Read the model definition and answer for the solid it produces. Units are mm, in the model's axes. A direction names the side the tool comes from. Coordinates: 2 decimals unless noted, no trailing zeros. Write each loop counter-clockwise with the first axis right and the second up, starting at its lowest first coordinate (ties: lowest second). Pieces come first, ordered by that corner, then holes.
Item 1: Section C-C (z = -1.75) is taken. Give the vertices of the cut face in (x, y), then the cut area to 3 significant figures.
Item 2: Section A-A (y = -8.8) is taken. Give the vertices of the cut face in (x, z).
Item 3: Section B-B (x = -16) is taken. Give the vertices of the cut face in (y, z), then the cut area to 3 significant figures.
Item 4: A tool of negligible diameter and unlimited length cuts with its end or side. For faces 4 (the face through (-10.964, -8, 4)), 5 (the face through (-28, -8, 0.2)), 6 (the face through (-22.964, -8, -3)), 7 (the face through (-20, -10.457, -3)), 8 (the face through (-20, -6.257, -3)), from which of +Z, -Z, +X, -X, +Y, -Y can it reach the whole face along a straight path? Write none if from no direction.
Item 5: Straight lines are drawn through the part: probe 1 along X at (y, z) = (-8.3, 6.75); probe 2 along X at (y, z) = (-6.75, -2.5); probe 3 along Z at (x, y) = (-17.5, -7.2). For each, find the intervals that lie inside material, in ascending order.
Item 6: Each of these flat-tipped pins is pushed along its axis until it touches: P1, Ø2, axis at x = -9.5, y = -8, coming from the +Z side; P2, Ø2, axis at y = -7.5, z = -3, coming from the +X side; P3, Ø4, axis at x = -21.5, z = -1.5, coming from the -Y side; P4, Ø3, axis at y = -7.5, z = 4, coming from the +X side. Where does it stop, or does it pass through?
Item 7: Section D-D (x = -20.5) is taken. Give the vertices of the cut face in (y, z), then the cut area to 3 significant figures.
Item 8: Determine the mould class of faces 1 (the face through (-16, -8, 0.2)), 2 (the face through (-25.964, -8, 4)), 3 (the face through (-9, -8, 0.2)) for opening direction X: released by +X, released by -X, zero draft, split by the parting line, or undercut.
from build123d import *

# Parameters (mm, degrees)
F0_W     = 23
F0_H     = 6
F1_DEPTH = 0.2
F2_W     = 15
F2_H     = 6
F3_DEPTH = 7
F4_W     = 9
F4_H     = 4.2
F5_DEPTH = 0.2
F6_W     = 5
F6_H     = 4.2
F7_DEPTH = 5.3


with BuildPart() as f1:
    # F0 (on Top) → F1 (new body)
    with BuildSketch(Plane.XY):
        with Locations((-18.463512, -8.357231)):
            Rectangle(F0_W, F0_H)
    extrude(amount=F1_DEPTH)

    # F2 (on face) → F3 (join)
    with BuildSketch(Plane.XY.offset(0.2)):
        with Locations((-18.463512, -8.357231)):
            Rectangle(F2_W, F2_H)
    extrude(amount=F3_DEPTH)

    # F4 (on face) → F5 (cut)
    with BuildSketch(Plane(origin=(0, 0, 0), x_dir=(1, 0, 0), z_dir=(0, 0, -1))):
        with Locations((-18.463512, 8.357231)):
            Rectangle(F4_W, F4_H)
    extrude(amount=-F5_DEPTH, mode=Mode.SUBTRACT)

    # F6 (on face) → F7 (join)
    with BuildSketch(Plane(origin=(0, 0, 0.2), x_dir=(1, 0, 0), z_dir=(0, 0, -1))):
        with Locations((-20.463512, 8.357231)):
            Rectangle(F6_W, F6_H)
    extrude(amount=F7_DEPTH)


solid = f1.part
Established:
1. outline: (-22.96, -10.46) - (-17.96, -10.46) - (-17.96, -6.26) - (-22.96, -6.26) - close
1. area: 21.0 mm2
2. outline: (-29.96, 0) - (-22.96, 0) - (-22.96, -5.1) - (-17.96, -5.1) - (-17.96, 0.2) - (-13.96, 0.2) - (-13.96, 0) - (-6.96, 0) - (-6.96, 0.2) - (-10.96, 0.2) - (-10.96, 7.2) - (-25.96, 7.2) - (-25.96, 0.2) - (-29.96, 0.2) - close
3. outline: (-11.36, 0) - (-10.46, 0) - (-10.46, 0.2) - (-6.26, 0.2) - (-6.26, 0) - (-5.36, 0) - (-5.36, 7.2) - (-11.36, 7.2) - close
3. area: 42.4 mm2
4. face 4: +Z, +X, +Y, -Y
4. face 5: +Z, -X, +Y, -Y
4. face 6: -Z, -X, +Y, -Y
4. face 7: -Z, +X, -X, -Y
4. face 8: -Z, +X, -X, +Y
5. probe 1: x = -25.96 to -10.96
5. probe 2: x = -22.96 to -17.96
5. probe 3: z = 0.2 to 7.2
6. P1: stops at z = 0.2
6. P2: stops at x = -17.96
6. P3: stops at y = -11.36
6. P4: stops at x = -10.96
7. outline: (-11.36, 0) - (-10.46, 0) - (-10.46, -5.1) - (-6.26, -5.1) - (-6.26, 0) - (-5.36, 0) - (-5.36, 7.2) - (-11.36, 7.2) - close
7. area: 64.6 mm2
8. face 1: undercut
8. face 2: released by -X
8. face 3: zero draft
